For this review, take the finished solid that the model builds, in its own axes (mm). A direction names the side the tool comes from. Give positions to 0.01 mm unless a question says otherwise; leave off trailing zeros. Loops run counter-clockwise (first coordinate to the right, second up) from the corner with the lowest first, then second, coordinate; pieces in that order, holes last. Notation, with made-up numbers: M 25,-35 L 73,-35 A18 cw 73,-17 Z; hole C -35,-28 d4. An arc over 180 degrees is marked long. Use CSV: the item, a comma, the result in double quotes. Start each with the question number.
1. Insertion check: P1, Ø5, axis at y = -94.5, z = 3, coming from the +X side; P2, Ø3, axis at x = 3, z = 5.5, coming from the +Y side; P3, Ø6, axis at y = -67, z = 1, coming from the -X side; P4, Ø5, axis at y = -92.5, z = 6.5, coming from the -X side. Each pin has a flat end and moves straight along its axis. Give the tip position at first contact, or say it passes through.
2. Take a section at B-B, the plane y = -90. Write out the cut boundary in (x, z), and give its area (3 significant figures).
3. Take a section at A-A, the plane z = 5.25. Write out the cut boundary in (x, y).
4. Take a section at C-C, the plane x = 93. Write out the cut boundary in (y, z).
5. To check wall thickness, follow line 1 (X direction, y = -91, z = 3.75); line 2 (Y direction, x = 9, z = 7.5). State the ranges of each line that lie inside material, in increasing order. Write a range as [from, to].
6. Tool access review of faces 1 (the face through (6, -12, 5)), 2 (the face through (94, -12, 5)), 3 (the face through (6, -88, 5)), 4 (the face through (94, -88, 5)), 5 (the face through (100, -51, 5)): name each direction out of +Z, -Z, +X, -X, +Y, -Y from which nothing blocks a thin tool from reaching the whole face with its end or side.
from build123d import *

# Parameters (mm, degrees)
F0_W     = 500
F0_H     = 500
F1_DEPTH = 50
F2_W     = 60
F2_H     = 60
F3_DEPTH = 90
F4_SCALE = 0.2


with BuildPart() as f1:
    # F0 (on Top) → F1 (new body)
    with BuildSketch(Plane.XY):
        with Locations((250, -250)):
            Rectangle(F0_W, F0_H)
    extrude(amount=F1_DEPTH)

    # F2 (on face) → F3 (cut)
    with BuildSketch(Plane.XY.offset(50)):
        with Locations((470, -470)):
            Rectangle(F2_W, F2_H)
        with Locations((30, -30)):
            Rectangle(F2_W, F2_H)
        with Locations((30, -470)):
            Rectangle(F2_W, F2_H)
        with Locations((470, -30)):
            Rectangle(F2_W, F2_H)
    extrude(amount=-F3_DEPTH, mode=Mode.SUBTRACT)


with BuildPart() as f1_1:
    # F4: moved
    add(f1.part.scale(F4_SCALE))


solid = f1_1.part
Result set:
1,P1,"x = 88"
1,P2,"y = -12"
1,P3,"x = 0"
1,P4,"x = 12"
2,outline,"M 12,0 L 88,0 L 88,10 L 12,10 Z"
2,area,"760 mm2"
3,outline,"M 0,-88 L 12,-88 L 12,-100 L 88,-100 L 88,-88 L 100,-88 L 100,-12 L 88,-12 L 88,0 L 12,0 L 12,-12 L 0,-12 Z"
4,outline,"M -88,0 L -12,0 L -12,10 L -88,10 Z"
5,line 1,"[12, 88]"
5,line 2,"[-88, -12]"
6,face 1,"+Z, -Z, -X, +Y"
6,face 2,"+Z, -Z, +X, +Y"
6,face 3,"+Z, -Z, -X, -Y"
6,face 4,"+Z, -Z, +X, -Y"
6,face 5,"+Z, -Z, +X, +Y, -Y"
